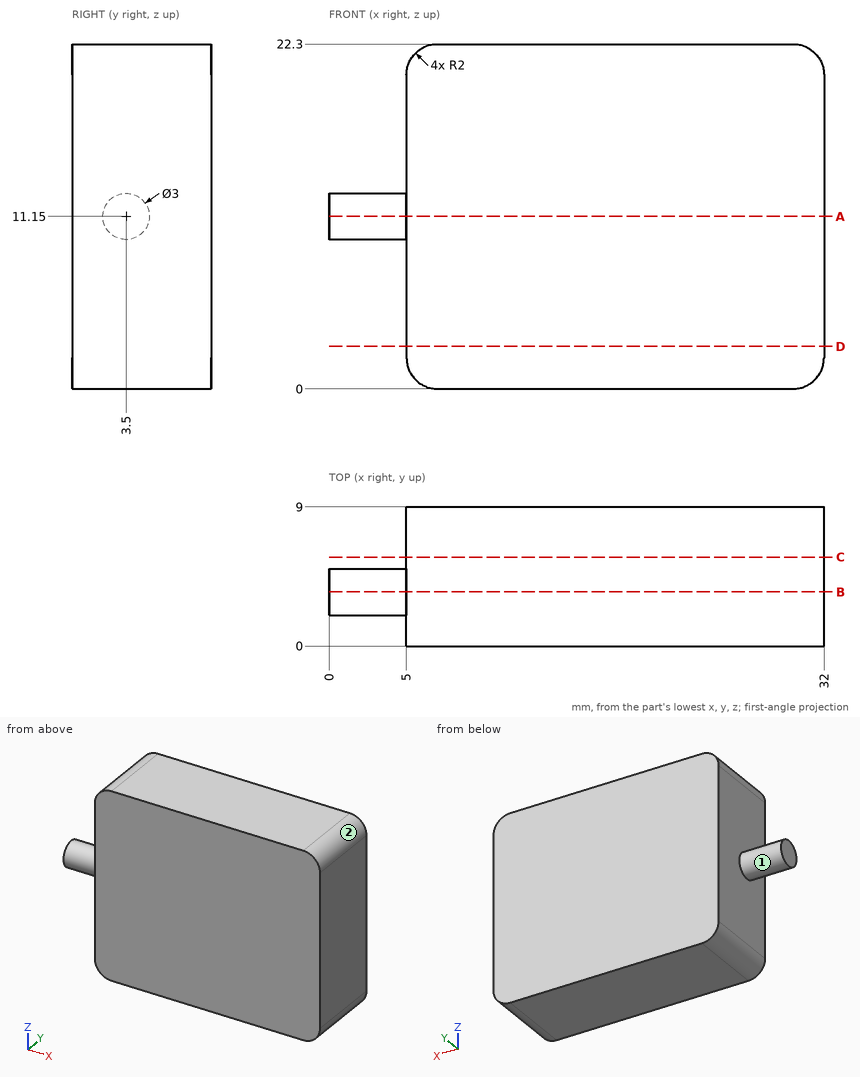
Print and shaded views of the part. All mm, measured from the part's lowest x, y and z. A direction names the side the tool comes from. Round coordinates to 2 decimals unless told otherwise and drop trailing zeros. Write each loop counter-clockwise with the first axis right and the second up, starting at its lowest first coordinate (ties: lowest second). Pieces come first, ordered by that corner, then holes. Notation, with made-up numbers: (-33.75, 14) - (-19.75, 14) arc R16 ccw to (-19.75, 26) - close; hole circle Ø7 at (-9.5, 76). An arc over 180 degrees is marked (long way). Use CSV: the item, a comma, the result in double quotes. Start each with the question number.
Item 1: Band-saw the part on A-A (z = 11.15). Write the cut outline in (x, y), and give its area (3 significant figures).
Item 2: Pin check, flat tips, straight feed: P1, Ø5, axis at x = 3.5, y = 6.5, coming from the +Z side; P2, Ø3, axis at y = 8, z = 15, coming from the -X side. Stop position of each tip, or through.
Item 3: Drill centre lines: L1, parallel to X at y = 6.5, z = 12.75; L2, parallel to X at y = 3, z = 1; L3, parallel to Z at x = 31, y = 6.75. Where is each one in solid material? Low to high. Write a range as [from, to].
Item 4: Band-saw the part on C-C (y = 5.75). Write the cut outline in (x, z).
Item 5: Band-saw the part on B-B (y = 3.5). Write the cut outline in (x, z).
Item 6: Tool access for the marked faces 1 and 2: list every direction of +Z, -Z, +X, -X, +Y, -Y with a clear straight run to the whole face (end or side of a thin tool).
Item 7: Band-saw the part on D-D (z = 2.75). Write the cut outline in (x, y).
Checked values:
1,outline,"(0, 2) - (5, 2) - (5, 0) - (32, 0) - (32, 9) - (5, 9) - (5, 5) - (0, 5) - close"
1,area,"258 mm²"
2,P1,"stops at z = 22.03"
2,P2,"stops at x = 5"
3,L1,"x = [5, 32]"
3,L2,"x = [5.27, 31.73]"
3,L3,"z = [0.27, 22.03]"
4,outline,"(5, 2) arc R2 ccw to (7, 0) - (30, 0) arc R2 ccw to (32, 2) - (32, 20.3) arc R2 ccw to (30, 22.3) - (7, 22.3) arc R2 ccw to (5, 20.3) - close"
5,outline,"(0, 9.65) - (5, 9.65) - (5, 2) arc R2 ccw to (7, 0) - (30, 0) arc R2 ccw to (32, 2) - (32, 20.3) arc R2 ccw to (30, 22.3) - (7, 22.3) arc R2 ccw to (5, 20.3) - (5, 12.65) - (0, 12.65) - close"
6,face 1,"-X"
6,face 2,"+Z, +X, +Y, -Y"
7,outline,"(5, 0) - (32, 0) - (32, 9) - (5, 9) - close"
